Geometry check sheet. Reference: the model listing, model coordinates, mm. A direction names the side the tool comes from. Coordinates: 2 decimals unless noted, no trailing zeros. Write each loop counter-clockwise with the first axis right and the second up, starting at its lowest first coordinate (ties: lowest second). Pieces come first, ordered by that corner, then holes. Notation, with made-up numbers: M 54.25,38 L 80.25,38 A9 cw 80.25,48 Z; hole C -23.75,64 d4. An arc over 180 degrees is marked long. Answer as a JSON object with one key per item and string values. Group by question number.
```python
from build123d import *

# Parameters (mm, degrees)
SKETCH1_W           = 73
SKETCH1_H           = 34.25
BOSS_EXTRUDE1_DEPTH = 4.5
FILLET1_R           = 2
SKETCH2_W           = 70.1
SKETCH2_H           = 32.1
SKETCH2_W_2         = 68.1
SKETCH2_H_2         = 30.1
BOSS_EXTRUDE2_DEPTH = 2
SKETCH3_W           = 68.1
SKETCH3_H           = 30.1
CUT_EXTRUDE1_DEPTH  = 3


with BuildPart() as part:
    # Sketch1 → Boss-Extrude1 (new body)
    with BuildSketch(Plane(origin=(0, 0, 0), x_dir=(1, 0, 0), z_dir=(0, 1, 0))):
        with Locations((-0.414772727, -1.263257576)):
            Rectangle(SKETCH1_W, SKETCH1_H)
    extrude(amount=BOSS_EXTRUDE1_DEPTH)

    # Fillet1
    fillet1_edges = [part.edges().sort_by_distance(p)[0] for p in [
        (-36.914772727, 2.25, -15.861742424),
        (36.085227273, 2.25, -15.861742424),
        (36.085227273, 2.25, 18.388257576),
        (-36.914772727, 2.25, 18.388257576),
    ]]
    fillet(fillet1_edges, radius=FILLET1_R)

    # Sketch2 → Boss-Extrude2 (add)
    with BuildSketch(Plane(origin=(0, 4.5, 0), x_dir=(1, 0, 0), z_dir=(0, 1, 0))):
        with Locations((-0.414772727, -0.888257576)):
            Rectangle(SKETCH2_W, SKETCH2_H)
        with Locations((-0.414772727, -0.888257576)):
            Rectangle(SKETCH2_W_2, SKETCH2_H_2, mode=Mode.SUBTRACT)
    extrude(amount=BOSS_EXTRUDE2_DEPTH)

    # Sketch3 → Cut-Extrude1 (cut)
    with BuildSketch(Plane(origin=(0, 4.5, 0), x_dir=(1, 0, 0), z_dir=(0, 1, 0))):
        with Locations((-0.414772727, -0.888257576)):
            Rectangle(SKETCH3_W, SKETCH3_H)
    extrude(amount=-CUT_EXTRUDE1_DEPTH, mode=Mode.SUBTRACT)


solid = part.part
```
1) Set-up check for faces 1 (the flat face through (-1, 4, -14.162)), 2 (the flat face through (-1, 5, -15.162)), 3 (the flat face through (34.635, 5, 1)): record each of +Z, -Z, +X, -X, +Y, -Y from which the full face is reachable in a straight line by a thin tool's end or side.
2) Section check B-B (z = 14.5). Record the cut outline in (x, y), then the cut area to 3 significant figures.
3) Section check C-C (x = 12.5). Record the cut outline in (y, z), then the cut area to 3 significant figures.
4) Go/stop test with flat-tipped pins: pin 1 Ø0.6 at (x, y) = (-5, 6) entering from +Z; pin 2 Ø1.6 at (x, y) = (12.5, 5.5) entering from -Z; pin 3 Ø9 at (x, z) = (-9.5, 1.5) entering from +Y. Record where each tip stops, or that it passes through.
5) Section check A-A (y = 3.75). Record the cut outline in (x, z).
6) Draft check along X on faces 4 (the cylindrical face through (35.515, 2.282, -15.26)), 5 (the flat face through (-34.465, 4, 1)), 6 (the flat face through (-11, 4.5, 18)). Enter one of: +X half, -X half, draft (parallel to the pull), parting line (faces both ways), or undercut.
7) Material ranges on probe 1 along Z at (x, y) = (5, 5.5); probe 2 along X at (y, z) = (5.75, -13.5); probe 3 along X at (y, z) = (2.5, 3), recorded low to high. Write a range as [from, to].
Entries:
{
 "1": {"face 1": "+Y", "face 2": "-Z, +X, -X, +Y", "face 3": "+Z, -Z, +X, +Y"},
 "2": {"outline": "M -36.91,0 L 36.09,0 L 36.09,4.5 L 34.64,4.5 L 34.64,6.5 L 33.64,6.5 L 33.64,1.5 L -34.46,1.5 L -34.46,6.5 L -35.46,6.5 L -35.46,4.5 L -36.91,4.5 Z", "area": "128 mm^2"},
 "3": {"outline": "M 0,-15.86 L 4.5,-15.86 L 4.5,-15.16 L 6.5,-15.16 L 6.5,-14.16 L 1.5,-14.16 L 1.5,15.94 L 6.5,15.94 L 6.5,16.94 L 4.5,16.94 L 4.5,18.39 L 0,18.39 Z", "area": "67.8 mm^2"},
 "4": {"pin 1": "z = 16.94", "pin 2": "z = -15.16", "pin 3": "y = 1.5"},
 "5": {"outline": "M -36.91,-13.86 A2 ccw -34.91,-15.86 L 34.09,-15.86 A2 ccw 36.09,-13.86 L 36.09,16.39 A2 ccw 34.09,18.39 L -34.91,18.39 A2 ccw -36.91,16.39 Z; hole M -34.46,-14.16 L 33.64,-14.16 L 33.64,15.94 L -34.46,15.94 Z"},
 "6": {"face 4": "+X half", "face 5": "undercut", "face 6": "draft"},
 "7": {"probe 1": "[-15.16, -14.16], [15.94, 16.94]", "probe 2": "[-35.46, -34.46], [33.64, 34.64]", "probe 3": "[-36.91, -34.46], [33.64, 36.09]"}
}
